Solid Edge part; units mm, degrees
sketch "Sketch1" plane through (0, 0, 0) normal (0, 0, 1) x (1, 0, 0)
  line L0 (-30, -30) -> (30, -30)
  line L1 (30, -30) -> (30, 30)
  line L2 (30, 30) -> (-30, 30)
  line L3 (-30, 30) -> (-30, -30)
  dimension "D1" = 30
  dimension "D2" = 30
extrude "Protrusion1" add sketch "Sketch1" along normal blind 2
fillet "Congé_1" radius 1.9 4 edges at (30, -30, 1) (-30, -30, 1) (30, 30, 1) (-30, 30, 1)
sketch "Sketch2" plane through (0, 0, 2) normal (0, 0, 1) x (1, 0, 0)
  circle A0 centre (-25, 25) radius 2.1
  circle A1 centre (-25, -25) radius 2.1
  circle A2 centre (25, -25) radius 2.1
  circle A3 centre (25, 25) radius 2.1
  dimension "D1" = 25
extrude "Cutout1" cut sketch "Sketch2" against normal up to next
Could you check a few things on this model? Use its own coordinates, in mm. Coordinates: 2 decimals unless noted, no trailing zeros. Loops run counter-clockwise (first coordinate to the right, second up) from the corner with the lowest first, then second, coordinate; pieces in that order, holes last.
1. Imagine slicing it at A-A (x = 25). Please give me the cut outline in (y, z).
2. We'd pull the mould along Y, two halves only. Please class faces 1 (the face through (27.003, 25.631, 1.014)), 2 (the face through (-29.458, -29.429, 1.014)), 3 (the face through (29.458, 29.429, 1.014)): released by +Y, released by -Y, zero draft, split by the parting line, or undercut.
3. I need wall thicknesses on L1, parallel to Y at x = -25, z = 1.5; L2, parallel to X at y = -23.5, z = 1.6; L3, parallel to Y at x = -24.5, z = 1.1. Which ranges of each line are inside material? Lowest first, please.
4. Imagine slicing it at B-B (z = 1). Please give me the cut outline in (x, y).
Computed values:
1. outline: (-30, 0) - (-27.1, 0) - (-27.1, 2) - (-30, 2) - close; (-22.9, 0) - (22.9, 0) - (22.9, 2) - (-22.9, 2) - close; (27.1, 0) - (30, 0) - (30, 2) - (27.1, 2) - close
2. face 1: undercut
2. face 2: released by -Y
2. face 3: released by +Y
3. L1: y = -30 to -27.1, -22.9 to 22.9, 27.1 to 30
3. L2: x = -30 to -26.47, -23.53 to 23.53, 26.47 to 30
3. L3: y = -30 to -27.04, -22.96 to 22.96, 27.04 to 30
4. outline: (-30, -28.1) arc R1.9 ccw to (-28.1, -30) - (28.1, -30) arc R1.9 ccw to (30, -28.1) - (30, 28.1) arc R1.9 ccw to (28.1, 30) - (-28.1, 30) arc R1.9 ccw to (-30, 28.1) - close; hole circle Ø4.2 at (-25, -25); hole circle Ø4.2 at (-25, 25); hole circle Ø4.2 at (25, -25); hole circle Ø4.2 at (25, 25)
